Can you work these out from the model? Positions are in its coordinate system, mm. Face numbers are marked on the shaded views. A direction names the side the tool comes from. Round coordinates to 2 decimals unless told otherwise and drop trailing zeros. Loops run counter-clockwise (first coordinate to the right, second up) from the corner with the lowest first, then second, coordinate; pieces in that order, holes last. Notation, with made-up numbers: M 4,47.25 L 26,47.25 A8 ccw 26,51.25 Z; hole C -32,-17.5 d7. An arc over 180 degrees is marked long. Answer as CSV lines item,"result".
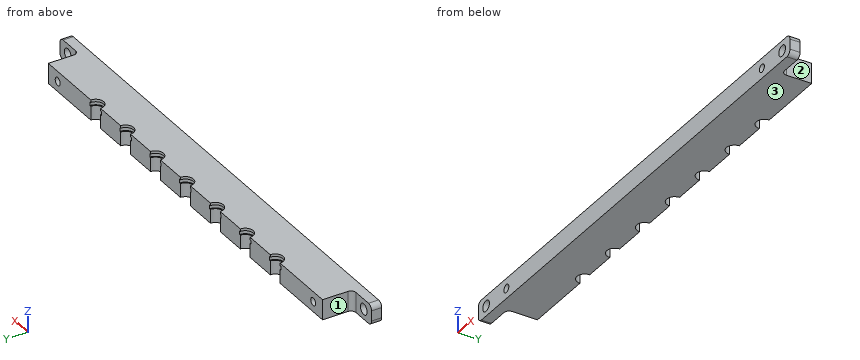
from build123d import *

# Parameters (mm, degrees)
SKETCH1_W                   = 139.7
SKETCH1_H                   = 12.7
BOSS_EXTRUDE1_DEPTH         = 6.35
TAP_DRILL_FOR_M3X0_5_TAP1_D = 2.5
SKETCH5_W                   = 9.525
SKETCH5_H                   = 6.35
BOSS_EXTRUDE2_DEPTH         = 3.175
FILLET1_R                   = 1.5875
M3_CLEARANCE_HOLE1_D        = 3.4
FILLET2_R                   = 1.5875
FILLET2_OF_MIRROR5_R        = 1.5875
FILLET3_R                   = 1.5875
SKETCH14_R                  = 2.5
CUT_EXTRUDE2_DEPTH          = 0.79375
SKETCH15_R                  = 2.921
CUT_EXTRUDE3_DEPTH          = 1.2065
CUT_EXTRUDE4_START          = -5.34975
CUT_EXTRUDE4_DEPTH          = 8.35
LPATTERN1_COUNT             = 4
LPATTERN1_PITCH             = 15.24
LPATTERN2_COUNT             = 4
LPATTERN2_PITCH             = 15.24


with BuildPart() as part:
    # Sketch1 → Boss-Extrude1 (new body)
    with BuildSketch(Plane.XY):
        Rectangle(SKETCH1_W, SKETCH1_H)
    extrude(amount=BOSS_EXTRUDE1_DEPTH)

    # Tap Drill for M3x0.5 Tap1 (through all)
    with Locations(Plane(origin=(0, 6.35, 0), x_dir=(1, 0, 0), z_dir=(0, 1, 0))):
        with Locations((-65.0875, -3.175), (65.0875, -3.175)):
            Hole(TAP_DRILL_FOR_M3X0_5_TAP1_D / 2)

    # Sketch5 → Boss-Extrude2 (add)
    with BuildSketch(Plane.XZ.offset(6.35)):
        with Locations((-74.6125, 3.175)):
            Rectangle(SKETCH5_W, SKETCH5_H)
    boss_extrude2 = extrude(amount=-BOSS_EXTRUDE2_DEPTH)

    # Fillet1
    fillet1_edges = [part.edges().sort_by_distance(p)[0] for p in [
        (-69.85, -3.175, 3.175),
    ]]
    fillet(fillet1_edges, radius=FILLET1_R)

    # M3 Clearance Hole1 (through all)
    with Locations(Plane(origin=(0, -3.175, 0), x_dir=(1, 0, 0), z_dir=(0, 1, 0))):
        with Locations((-75.40625, -3.175)):
            m3_clearance_hole1 = Hole(M3_CLEARANCE_HOLE1_D / 2)

    # Fillet2
    fillet2_edges = [part.edges().sort_by_distance(p)[0] for p in [
        (-79.375, -4.7625, 0),
        (-79.375, -4.7625, 6.35),
    ]]
    fillet(fillet2_edges, radius=FILLET2_R)

    # Mirror5: Boss-Extrude2, M3 Clearance Hole1 across plane
    add(boss_extrude2.mirror(Plane(origin=(0, 0, 0), x_dir=(0, 0, 1), z_dir=(1, 0, 0))))
    add(m3_clearance_hole1.mirror(Plane(origin=(0, 0, 0), x_dir=(0, 0, 1), z_dir=(1, 0, 0))), mode=Mode.SUBTRACT)

    # Fillet2 of Mirror5
    fillet2_of_mirror5_edges = [part.edges().sort_by_distance(p)[0] for p in [
        (79.375, -4.7625, 0),
        (79.375, -4.7625, 6.35),
    ]]
    fillet(fillet2_of_mirror5_edges, radius=FILLET2_OF_MIRROR5_R)

    # Fillet3
    fillet3_edges = [part.edges().sort_by_distance(p)[0] for p in [
        (69.85, -3.175, 3.175),
    ]]
    fillet(fillet3_edges, radius=FILLET3_R)

    # Sketch14 → Cut-Extrude2 (cut)
    with BuildSketch(Plane.XY.offset(6.35)):
        with Locations((0, 6.35)):
            Circle(SKETCH14_R)
    cut_extrude2 = extrude(amount=-CUT_EXTRUDE2_DEPTH, mode=Mode.SUBTRACT)

    # Sketch15 → Cut-Extrude3 (cut)
    with BuildSketch(Plane.XY.offset(5.55625)):
        with Locations((0, 6.35)):
            Circle(SKETCH15_R)
    cut_extrude3 = extrude(amount=-CUT_EXTRUDE3_DEPTH, mode=Mode.SUBTRACT)

    # Sketch16 → Cut-Extrude4 (cut)
    with BuildSketch(Plane.XY.offset(4.34975).offset(CUT_EXTRUDE4_START)):
        with BuildLine():
            Line((-2.5, 182.058245118), (-2.5, 6.35))
            ThreePointArc((-2.5, 6.35), (0, 3.85), (2.5, 6.35))
            Line((2.5, 6.35), (2.5, 182.058245118))
            Line((2.5, 182.058245118), (2.5, 533.474735353))
            Line((2.5, 533.474735353), (-2.5, 533.474735353))
            Line((-2.5, 533.474735353), (-2.5, 182.058245118))
        make_face()
    cut_extrude4 = extrude(amount=CUT_EXTRUDE4_DEPTH, mode=Mode.SUBTRACT)

    # LPattern1: Cut-Extrude2, Cut-Extrude3, Cut-Extrude4 ×4
    with Locations(*[(i * LPATTERN1_PITCH, 0, 0) for i in range(1, LPATTERN1_COUNT)]):
        add(cut_extrude2, mode=Mode.SUBTRACT)
        add(cut_extrude3, mode=Mode.SUBTRACT)
        add(cut_extrude4, mode=Mode.SUBTRACT)

    # LPattern2: Cut-Extrude2, Cut-Extrude3, Cut-Extrude4 ×4
    with Locations(*[(-i * LPATTERN2_PITCH, 0, 0) for i in range(1, LPATTERN2_COUNT)]):
        add(cut_extrude2, mode=Mode.SUBTRACT)
        add(cut_extrude3, mode=Mode.SUBTRACT)
        add(cut_extrude4, mode=Mode.SUBTRACT)


solid = part.part
Item 1: Will these pins go through, and if not, where does the flat tip stop? pin 1 (1.5 mm diameter, centred on x = -45.5, y = 5, fed in from +Z); pin 2 (1.9 mm diameter, centred on x = 75, z = 4.5, fed in from +Y) (3 decimals); pin 3 (1 mm diameter, centred on y = 2, z = 1.5, fed in from -X).
Output:
pin 1,"passes through"
pin 2,"stops at y = -3.175"
pin 3,"stops at x = -69.85"
Item 2: If we section it at A-A on x = -45.72: Write out the boundary of the cut face in (y, z), then the cut area to 3 significant figures.
Output:
outline,"M -6.35,0 L 3.85,0 L 3.85,4.35 L 3.43,4.35 L 3.43,5.56 L 3.85,5.56 L 3.85,6.35 L -6.35,6.35 Z"
area,"64.3 mm2"
Item 3: If I drill on line 1 along X through (y, z) = (1, 4.25); line 2 along X through (y, z) = (1.25, 4); line 3 along X through (y, z) = (-0.25, 5), over which ranges is the centre line in solid material (lowest first)? Write a range as from..to.
Output:
line 1,"x = -69.85..-65.73, -64.45..64.45, 65.73..69.85"
line 2,"x = -69.85..-66.03, -64.15..64.15, 66.03..69.85"
line 3,"x = -69.85..69.85"
Item 4: On a 3-axis mill with a long thin cutter (end or side, diameter ignored), from which of +Z, -Z, +X, -X, +Y, -Y can I reach the whole of each face in a straight line? I mean the marked faces 1, 2 and 3. Say none if no direction works.
Output:
face 1,"+Z, -Z, -X, +Y"
face 2,"+Z, -Z, +X, +Y"
face 3,"-Z, +X, -X, +Y, -Y"
Item 5: If we section it at B-B on y = 0: State how many separate pieces and enclosed holes the cut face has, then the cut area to 3 significant figures.
Output:
separate pieces,"1"
enclosed holes,"2"
area,"877 mm2"
